The listing builds one solid part. Answer for the finished solid, in the listing's coordinates (mm). A direction names the side the tool comes from. Coordinates: 2 decimals unless noted, no trailing zeros. Loops run counter-clockwise (first coordinate to the right, second up) from the corner with the lowest first, then second, coordinate; pieces in that order, holes last. Notation, with made-up numbers: M -30,9.5 L -6,9.5 A29 cw -6,37.5 Z; hole C 64.5,-11.75 d10. An arc over 180 degrees is marked long. Return JSON: item names as keys, results as strings. Group by question number.
1. Section B-B (x = -305.5) is taken. Write down the section's boundary in (y, z).
2. The mould has two halves that part along Y. Classify faces 4 (the face through (-270, 128, 0)), 5 (the face through (-227.88, 40.597, 4.202)), 6 (the face through (-244, 123.759, 4)): pulls with the +Y half, pulls with the -Y half, needs draft (parallel to the pull), parting line crosses it, or undercut.
3. Section A-A (z = 4) is taken. Write down the section's boundary in (x, y), then the cut area to 3 significant figures.
4. Which of the six approach directions +Z, -Z, +X, -X, +Y, -Y give full straight-line access (tool end or side, diameter ignored) to faces 1 (the face through (-305, 123.759, 4)), 2 (the face through (-269, 132.259, 4)), 3 (the face through (-234.59, 84.72, 4.2))?
5. Given P1, Ø0.9, axis at x = -229.5, y = 41.5, coming from the -Z side; P2, Ø4, axis at x = -307.5, z = 3.5, coming from the -Y side; P3, Ø5, axis at x = -295, z = 4.5, coming from the -Y side; P4, Ø10, axis at x = -257, y = 91, coming from the +Z side, each flat-ended and moving along its own axis, determine where each tip first touches the part or whether it passes through.
6. Straight lines are drawn through the part: L1, parallel to Y at x = -240, z = 7.5; L2, parallel to Y at x = -265.5, z = 7.25; L3, parallel to Y at x = -239.5, z = 3.5. For each, find the intervals that lie inside material, in ascending order. Write a range as from..to.
```python
from build123d import *

# Parameters (mm, degrees)
BOSS_EXTRU_1_DEPTH           = 8.5
CONG_1_R                     = 3
ENL_V_MAT_EXTRU_1_DEPTH      = 75
ENL_V_MAT_EXTRU_1_DEPTH_BACK = 75


with BuildPart() as part:
    # Esquisse1 → Boss.-Extru.1 (new body)
    with BuildSketch(Plane.XY):
        with BuildLine():
            Line((-224.585732, 132.259189), (-314.419566, 132.259189))
            Line((-314.419566, 132.259189), (-314.419566, 123.759189))
            Line((-314.419566, 123.759189), (-294.419566, 123.759189))
            ThreePointArc((-294.419566, 123.759189), (-248.192676, 93.980686), (-231.088431, 41.720478))
            ThreePointArc((-231.088431, 41.720478), (-227.830568, 40.597512), (-224.585732, 41.757585))
            ThreePointArc((-224.585732, 41.757585), (-237.68722, 90.187689), (-274.970976, 123.759189))
            Line((-274.970976, 123.759189), (-224.585732, 123.759189))
            Line((-224.585732, 123.759189), (-224.585732, 132.259189))
        make_face()
    extrude(amount=BOSS_EXTRU_1_DEPTH)

    # Cong_1
    cong_1_edges = [part.edges().sort_by_distance(p)[0] for p in [
        (-274.970976, 123.759189, 4.25),
    ]]
    fillet(cong_1_edges, radius=CONG_1_R)

    # Esquisse2 → Enl_v. mat.-Extru.1 (cut, two sides)
    with BuildSketch(Plane(origin=(-224.585732, 0, 0), x_dir=(0, 0, -1), z_dir=(1, 0, 0))) as enl_v_mat_extru_1_sk:
        with BuildLine():
            Line((-8.5, 81.054434), (-8.5, 123.759189))
            add(Edge.make_bspline(
                [(-7.696596, 41.757585), (-4.874996, 82.844472), (-8.5, 123.759189)],
                knots=[0, 0, 0, 1, 1, 1], degree=2))
            Line((-7.696596, 41.757585), (-7.696596, 34.641133))
            Line((-7.696596, 34.641133), (-8.5, 34.641133))
            Line((-8.5, 34.641133), (-8.5, 81.054434))
        make_face()
        with BuildLine():
            Line((0, 123.759189), (0, 81.054434))
            Line((0, 81.054434), (0, 36.772624))
            Line((0, 36.772624), (-0.803404, 36.772624))
            Line((-0.803404, 36.772624), (-0.803404, 41.757585))
            add(Edge.make_bspline(
                [(-0.803404, 41.757585), (-3.625004, 82.844472), (0, 123.759189)],
                knots=[0, 0, 0, 1, 1, 1], degree=2))
        make_face()
    extrude(amount=ENL_V_MAT_EXTRU_1_DEPTH, mode=Mode.SUBTRACT)
    extrude(enl_v_mat_extru_1_sk.sketch, amount=-ENL_V_MAT_EXTRU_1_DEPTH_BACK, mode=Mode.SUBTRACT)


solid = part.part
```
Worked out:
{
 "1": {"outline": "M 123.76,0 L 132.26,0 L 132.26,8.5 L 123.76,8.5 Z"},
 "2": {"face 4": "needs draft", "face 5": "pulls with the -Y half", "face 6": "undercut"},
 "3": {"outline": "M -314.42,123.76 L -294.42,123.76 A82.19 cw -231.09,41.72 A5.2 ccw -224.59,41.76 A88.69 ccw -265.1,118.24 A3 cw -263.48,123.76 L -224.59,123.76 L -224.59,132.26 L -314.42,132.26 Z", "area": "1,480 mm^2"},
 "4": {"face 1": "+Z, -Z, -X, -Y", "face 2": "+Z, -Z, +X, -X, +Y", "face 3": "+Z, -Z, +X"},
 "5": {"P1": "z = 0.8", "P2": "y = 123.76", "P3": "y = 123.28", "P4": "through"},
 "6": {"L1": "123.76..132.26", "L2": "110.65..118.54, 122.97..132.26", "L3": "80.03..93.02, 123.76..132.26"}
}
